Can you work these out from the drawing? Everything is in mm from the part's minimum corner. A direction names the side the tool comes from. Coordinates: 2 decimals unless noted, no trailing zeros. Order: outer loops, then holes, each group sorted by start corner. A loop starts at its lowest first (then second) coordinate and runs counter-clockwise, first axis right, second up. Notation, with made-up numbers: (-19.75, 1) -> (35.25, 1) arc R29 ccw to (35.25, 21) -> close; hole circle Ø1 at (62.5, 37.25). An arc over 180 degrees is marked (long way). Return JSON: item names as keys, results as strings. Group by question number.
1) If we section it at A-A, the plane z = 1.5: Please give me the cut outline in (x, y).
2) If we section it at B-B, the plane x = 2.25: Please give me the cut outline in (y, z).
3) For the marked faces 4, 5 and 6, which set-ups out of +Z, -Z, +X, -X, +Y, -Y let a thin tool reach every point of the face, with its end or its side?
4) If we section it at D-D, the plane x = 4.5: Please give me the cut outline in (y, z).
5) If we section it at C-C, the plane y = 1.8: Please give me the cut outline in (x, z).
6) If I drill on probe 1 along X at (y, z) = (1.2, 1.5) (1 decimal); probe 2 along X at (y, z) = (1.4, 1.5); probe 3 along Z at (x, y) = (3.5, 1.3), over which ranges is the centre line in solid material (lowest first)? Write a range as from..to.
7) Thinking about a two-plate mould opening in X: for the marked faces 1, 2 and 3, which applies, +X half, -X half, draft (parallel to the pull), parting line (faces both ways), or undercut?
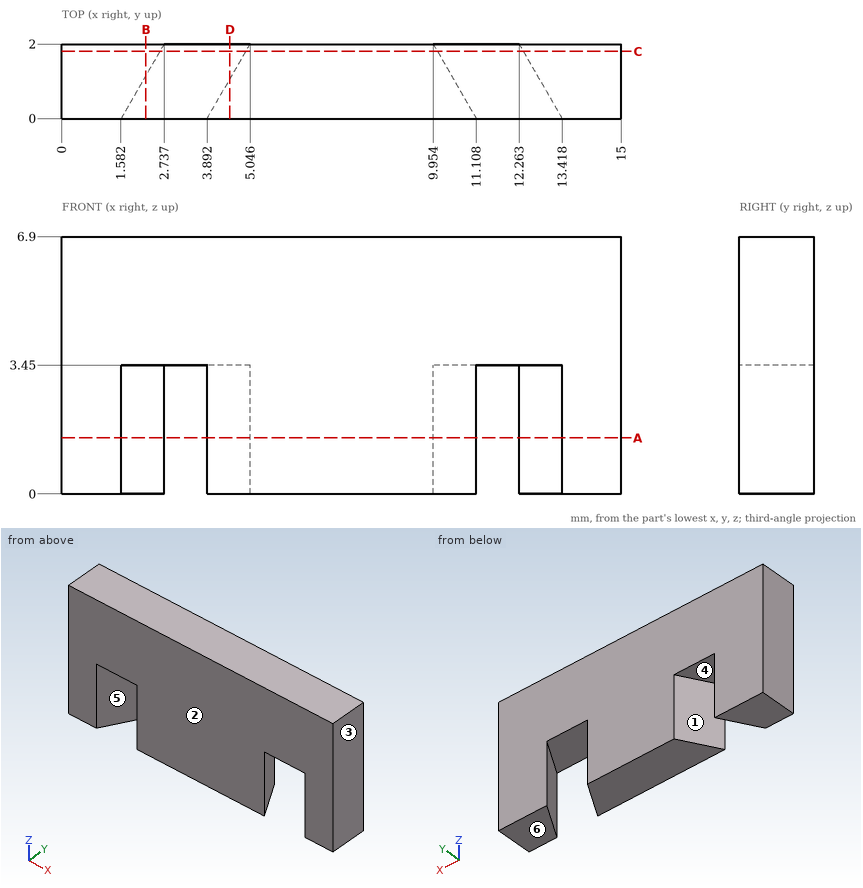
Result sheet:
{
 "1": {"outline": "(0, 0) -> (1.58, 0) -> (2.74, 2) -> (0, 2) -> close; (3.89, 0) -> (11.11, 0) -> (9.95, 2) -> (5.05, 2) -> close; (12.26, 2) -> (13.42, 0) -> (15, 0) -> (15, 2) -> close"},
 "2": {"outline": "(0, 3.45) -> (1.16, 3.45) -> (1.16, 0) -> (2, 0) -> (2, 6.9) -> (0, 6.9) -> close"},
 "3": {"face 4": "-Z", "face 5": "-Z, -Y", "face 6": "-Z, +X, -X, +Y, -Y"},
 "4": {"outline": "(0, 0) -> (1.05, 0) -> (1.05, 3.45) -> (2, 3.45) -> (2, 6.9) -> (0, 6.9) -> close"},
 "5": {"outline": "(0, 0) -> (2.62, 0) -> (2.62, 3.45) -> (4.93, 3.45) -> (4.93, 0) -> (10.07, 0) -> (10.07, 3.45) -> (12.38, 3.45) -> (12.38, 0) -> (15, 0) -> (15, 6.9) -> (0, 6.9) -> close"},
 "6": {"probe 1": "x = 0..2.3, 4.6..10.4, 12.7..15", "probe 2": "x = 0..2.39, 4.7..10.3, 12.61..15", "probe 3": "z = 3.45..6.9"},
 "7": {"face 1": "undercut", "face 2": "draft", "face 3": "+X half"}
}
